Can you work these out from the model? Positions are in its coordinate system, mm. Round coordinates to 2 decimals unless told otherwise and drop trailing zeros. Loops run counter-clockwise (first coordinate to the right, second up) from the corner with the lowest first, then second, coordinate; pieces in that order, holes last.
(1) If I drill on line 1 along Z through (x, y) = (0, 3); line 2 along X through (y, z) = (7.25, -0.75); line 3 along Z through (x, y) = (2.75, 1), over which ranges is the centre line in solid material (lowest first)?
(2) Thinking about a two-plate mould opening in Z: for faces 1 (the face through (-6.961, 4.856, 3.944)), 2 (the face through (4, 0, -4)), 3 (the face through (-1.08, 4.93, 4.88)), 4 (the face through (6.961, 4.856, -3.944)), which applies, released by +Z, released by -Z, zero draft, split by the parting line, or undercut?
(3) I want a section at A-A on x = 0. Write out the boundary of the cut face in (y, z), plus the area to 3 significant figures.
(4) Will these pins go through, and if not, where does the flat tip stop? pin 1 Ø9 at (x, z) = (0, 0) entering from +Y; pin 2 Ø6 at (y, z) = (1.5, 4.5) entering from +X; pin 3 Ø3 at (y, z) = (2, -6) entering from +X.
(5) I want a section at B-B on y = 2.5. Write out the boundary of the cut face in (x, z), plus the area to 3 significant figures.
from build123d import *

# Parameters (mm, degrees)
SKETCH1_R           = 5
BOSS_EXTRUDE1_DEPTH = 10


with BuildPart() as part:
    # Sketch1 → Boss-Extrude1 (new body)
    with BuildSketch(Plane(origin=(0, 0, 0), x_dir=(1, 0, 0), z_dir=(0, 1, 0))):
        Polygon((9.237604307, 0), (4.618802154, 8), (-4.618802154, 8), (-9.237604307, 0), (-4.618802154, -8), (4.618802154, -8), align=None)
        Circle(SKETCH1_R, mode=Mode.SUBTRACT)
    extrude(amount=BOSS_EXTRUDE1_DEPTH)

    # Sketch2 → Cut-Revolve1 (revolve, cut)
    with BuildSketch(Plane.XY):
        with BuildLine():
            Line((9.237604307, 10), (7.237604307, 10))
            ThreePointArc((7.237604307, 10), (8.651817869, 9.414213562), (9.237604307, 8))
            Line((9.237604307, 8), (9.237604307, 10))
        make_face()
    revolve(axis=Axis((0, 0, 0), (0, 1, 0)), mode=Mode.SUBTRACT)


solid = part.part
Filled sheet:
1. line 1: z = -8 to -5, 5 to 8
1. line 2: x = -8.8 to -4.94, 4.94 to 8.8
1. line 3: z = -8 to -4.18, 4.18 to 8
2. face 1: released by +Z
2. face 2: zero draft
2. face 3: undercut
2. face 4: released by -Z
3. outline: (0, -8) - (9.85, -8) arc R2 ccw to (10, -7.24) - (10, -5) - (0, -5) - close; (0, 5) - (10, 5) - (10, 7.24) arc R2 ccw to (9.85, 8) - (0, 8) - close
3. area: 59.9 mm2
4. pin 1: passes through
4. pin 2: stops at x = 8.37
4. pin 3: stops at x = 6.64
5. outline: (-9.24, 0) - (-4.62, -8) - (4.62, -8) - (9.24, 0) - (4.62, 8) - (-4.62, 8) - close; hole circle Ø10 at (0, 0)
5. area: 143 mm2
